The listing builds one solid part. Answer for the finished solid, in the listing's coordinates (mm). Face numbers are marked on the shaded views. A direction names the side the tool comes from. Round coordinates to 2 decimals unless told otherwise and drop trailing zeros. Write each loop counter-clockwise with the first axis right and the second up, starting at its lowest first coordinate (ties: lowest second). Pieces come first, ordered by that corner, then holes. Notation, with made-up numbers: (-11.75, 11.25) - (6.25, 11.25) arc R26 ccw to (6.25, 49.25) - close; hole circle Ø1 at (78, 87.5). An arc over 180 degrees is marked (long way). Answer in a Markdown table with one row per item.
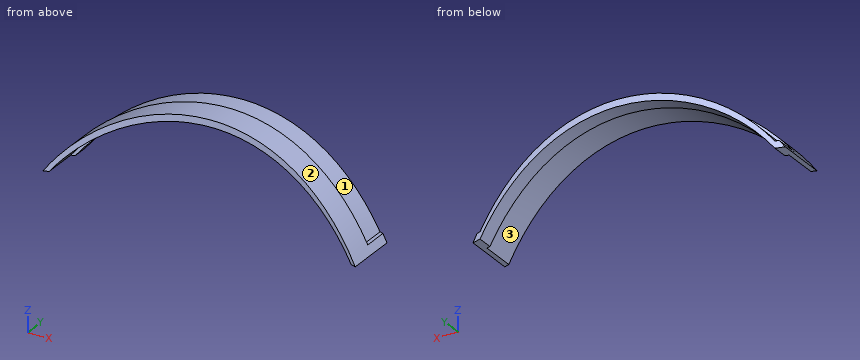
from build123d import *

# Parameters (mm, degrees)
PAD002_DEPTH    = 47.5
POCKET004_DEPTH = 67
POCKET005_DEPTH = 50
PAD001_DEPTH    = 47.5
POCKET002_DEPTH = 67
POCKET003_DEPTH = 50
PAD_DEPTH       = 47.5
POCKET_DEPTH    = 67
POCKET001_DEPTH = 50


with BuildPart() as body002:
    # Sketch006 → Pad002 (new body)
    with BuildSketch(Plane.XY):
        with BuildLine():
            ThreePointArc((90.501517, 0), (-0.00051, 14.750711), (-90.502537, 0))
            Line((-90.502537, 0), (-99.243083, 26.073989))
            ThreePointArc((99.233841, 26.076743), (-0.004846, 42.250711), (-99.243083, 26.073989))
            Line((90.501517, 0), (99.233841, 26.076743))
        make_face()
    extrude(amount=PAD002_DEPTH)

    # Sketch007 → Pocket004 (cut)
    with BuildSketch(Plane.XZ):
        with BuildLine():
            Line((0, 0), (-85.5, 0))
            ThreePointArc((85.5, 0), (0, 42.501931), (-85.5, 0))
            Line((0, 0), (85.5, 0))
        make_face()
    extrude(amount=-POCKET004_DEPTH, mode=Mode.SUBTRACT)

    # Sketch008 → Pocket005 (cut)
    with BuildSketch(Plane.XZ):
        with BuildLine():
            ThreePointArc((90.5, 0), (0, 47.5), (-90.5, 0))
            Line((-90.5, 0), (-105.5, 0))
            Line((-105.5, 0), (-105.5, 50))
            Line((-105.5, 50), (104.5, 50))
            Line((104.5, 50), (104.5, 0))
            Line((90.5, 0), (104.5, 0))
        make_face()
    extrude(amount=-POCKET005_DEPTH, mode=Mode.SUBTRACT)


with BuildPart() as body002_1:
    # Body002 placement: moved
    add(body002.part.moved(Location((0, 15, 4))))


with BuildPart() as body001:
    # Sketch003 → Pad001 (new body)
    with BuildSketch(Plane.XY):
        with BuildLine():
            ThreePointArc((90.501517, 0), (-0.00051, 14.750711), (-90.502537, 0))
            Line((-90.502537, 0), (-99.243083, 26.073989))
            ThreePointArc((99.233841, 26.076743), (-0.004846, 42.250711), (-99.243083, 26.073989))
            Line((90.501517, 0), (99.233841, 26.076743))
        make_face()
    extrude(amount=PAD001_DEPTH)

    # Sketch004 → Pocket002 (cut)
    with BuildSketch(Plane.XZ):
        with BuildLine():
            Line((0, 0), (-85.5, 0))
            ThreePointArc((85.5, 0), (0, 42.501931), (-85.5, 0))
            Line((0, 0), (85.5, 0))
        make_face()
    extrude(amount=-POCKET002_DEPTH, mode=Mode.SUBTRACT)

    # Sketch005 → Pocket003 (cut)
    with BuildSketch(Plane.XZ):
        with BuildLine():
            ThreePointArc((90.5, 0), (0, 47.5), (-90.5, 0))
            Line((-90.5, 0), (-105.5, 0))
            Line((-105.5, 0), (-105.5, 50))
            Line((-105.5, 50), (104.5, 50))
            Line((104.5, 50), (104.5, 0))
            Line((90.5, 0), (104.5, 0))
        make_face()
    extrude(amount=-POCKET003_DEPTH, mode=Mode.SUBTRACT)


with BuildPart() as body001_1:
    # Body001 placement: moved
    add(body001.part.moved(Location((0, -9, -4))))


with BuildPart() as cut001:
    # Sketch → Pad (new body)
    with BuildSketch(Plane.XY):
        with BuildLine():
            ThreePointArc((90.501517, 0), (-0.00051, 14.750711), (-90.502537, 0))
            Line((-90.502537, 0), (-99.243083, 26.073989))
            ThreePointArc((99.233841, 26.076743), (-0.004846, 42.250711), (-99.243083, 26.073989))
            Line((90.501517, 0), (99.233841, 26.076743))
        make_face()
    extrude(amount=PAD_DEPTH)

    # Sketch001 → Pocket (cut)
    with BuildSketch(Plane.XZ):
        with BuildLine():
            Line((0, 0), (-85.5, 0))
            ThreePointArc((85.5, 0), (0, 42.501931), (-85.5, 0))
            Line((0, 0), (85.5, 0))
        make_face()
    extrude(amount=-POCKET_DEPTH, mode=Mode.SUBTRACT)

    # Sketch002 → Pocket001 (cut)
    with BuildSketch(Plane.XZ):
        with BuildLine():
            ThreePointArc((90.5, 0), (0, 47.5), (-90.5, 0))
            Line((-90.5, 0), (-105.5, 0))
            Line((-105.5, 0), (-105.5, 50))
            Line((-105.5, 50), (104.5, 50))
            Line((104.5, 50), (104.5, 0))
            Line((90.5, 0), (104.5, 0))
        make_face()
    extrude(amount=-POCKET001_DEPTH, mode=Mode.SUBTRACT)

    # Cut: cut Body001
    add(body001_1.part, mode=Mode.SUBTRACT)

    # Cut001: cut Body002
    add(body002_1.part, mode=Mode.SUBTRACT)


solid = cut001.part
(1) Section B-B (y = 8) is taken. Give the vertices of the cut face in (x, z), and give its area (3 significant figures).
Checked values:
| item | result |
|---|---|
| outline | (-90.5, 0) - (-87.6, 0) arc R109.96 cw to (-61.66, 24.58) - (-61.66, 28.58) arc R109.96 ccw to start; (61.66, 24.58) arc R109.96 cw to (87.6, 0) - (90.5, 0) arc R109.96 ccw to (61.66, 28.58) - close |
| area | 219 mm2 |
(2) Flat-ended cylindrical pins translate along their axes: pin 1 (1.5 mm diameter, centred on x = 63.5, y = 19, fed in from +Z); pin 2 (0.6 mm diameter, centred on x = 86.5, y = 21.5, fed in from +Z); pin 3 (4 mm diameter, centred on y = 34, z = 40, fed in from +X). Find the tip coordinate at first contact, or state that the pin passes through.
Checked values:
| item | result |
|---|---|
| pin 1 | stops at z = 27.84 |
| pin 2 | stops at z = 4 |
| pin 3 | stops at x = 41.85 |
(3) Section A-A (z = 27.5) is taken. Give the vertices of the cut face in (x, y).
Checked values:
| item | result |
|---|---|
| outline | (-63.23, 7.65) arc R285.01 cw to (-57.12, 8.97) - (-57.12, 27.99) arc R312.51 cw to (-54.71, 28.43) - (-54.71, 37.43) arc R312.51 ccw to (-60.95, 36.25) - (-60.95, 23.16) arc R285.01 ccw to (-63.23, 22.65) - close; (54.71, 28.42) arc R312.51 cw to (57.12, 27.99) - (57.12, 8.97) arc R285.01 cw to (63.23, 7.65) - (63.23, 22.65) arc R285.01 ccw to (60.95, 23.16) - (60.95, 36.25) arc R312.51 ccw to (54.71, 37.42) - close |
(4) Section C-C (x = 68) is taken. Give the vertices of the cut face in (y, z).
Checked values:
| item | result |
|---|---|
| outline | (6.52, 19.95) - (25.76, 19.95) - (25.76, 18.19) - (34.76, 18.19) - (34.76, 22.19) - (21.52, 22.19) - (21.52, 23.95) - (6.52, 23.95) - close |
(5) Section D-D (z = 10) is taken. Give the vertices of the cut face in (x, y).
Checked values:
| item | result |
|---|---|
| outline | (-82.71, 2.49) arc R285.01 cw to (-79.03, 3.58) - (-79.03, 23.09) arc R312.51 cw to (-76.91, 23.64) - (-76.91, 32.64) arc R312.51 ccw to (-80.61, 31.68) - (-80.61, 18.12) arc R285.01 ccw to (-82.71, 17.49) - close; (76.91, 23.64) arc R312.51 cw to (79.03, 23.09) - (79.03, 3.58) arc R285.01 cw to (82.71, 2.49) - (82.71, 17.49) arc R285.01 ccw to (80.61, 18.11) - (80.61, 31.68) arc R312.51 ccw to (76.91, 32.64) - close |
(6) Find the intervals of material crossed by line 1 (X direction, y = 14, z = 11); line 2 (X direction, y = 9.5, z = 24); line 3 (Z direction, x = 2, y = 20.5), in increasing order.
Checked values:
| item | result |
|---|---|
| line 1 | x = -81.82 to -78.05, 78.05 to 81.82 |
| line 2 | x = -67.94 to -62.52, 62.52 to 67.94 |
| line 3 | z = 43.48 to 47.48 |
(7) For the marked faces 1, 2 and 3, determine the directions among +Z, -Z, +X, -X, +Y, -Y from which every point of the face is accessible in a straight line to the end or side of a thin tool.
Checked values:
| item | result |
|---|---|
| face 1 | +Z, +Y |
| face 2 | +Z, +Y, -Y |
| face 3 | -Z, -Y |
